CAD build for the part. Positions are in the model's coordinates, mm. Face numbers are marked on the shaded views. A direction names the side the tool comes from. Round coordinates to 2 decimals unless told otherwise and drop trailing zeros. Order: outer loops, then holes, each group sorted by start corner. A loop starts at its lowest first (then second) coordinate and runs counter-clockwise, first axis right, second up. Notation, with made-up numbers: (25.25, -23.75) -> (41.25, -23.75) arc R16 cw to (41.25, -1.75) -> close; hole circle Ø7 at (12, 26). An arc over 180 degrees is marked (long way). Return JSON: item names as keys, results as strings. Group by question number.
Q1. Cut at A-A (z = 6). Write the cut outline in (x, y).
Q2. Mould opens along Y. For the marked faces 1 and 2 say: +Y half, -Y half, draft (parallel to the pull), parting line (faces both ways), or undercut.
Q3. Probe line 1 along X through (y, z) = (10, 1.75); line 2 along X through (y, z) = (-25, 7.75). List the from-to ranges inside material, lowest first.
Q4. Flat gauge pins, fed straight in: pin 1 (1.8 mm diameter, centred on y = 28.5, z = 9.5, fed in from +X); pin 2 (8 mm diameter, centred on x = 26, y = -24, fed in from -Z); pin 3 (2 mm diameter, centred on y = 25, z = 7.5, fed in from +X); pin 4 (3 mm diameter, centred on x = -26, z = 12.5, fed in from +Y). Where does each tip first touch, or does it go through?
Q5. Which spindle directions (+Z, -Z, +X, -X, +Y, -Y) get a long thin tool onto all of the face, cutting with end or side? Do the marked faces 3 and 4. Say none if no direction does.
Q6. Cut at D-D (x = 28). Write the cut outline in (y, z).
Q7. Cut at B-B (x = -8). Write the cut outline in (y, z).
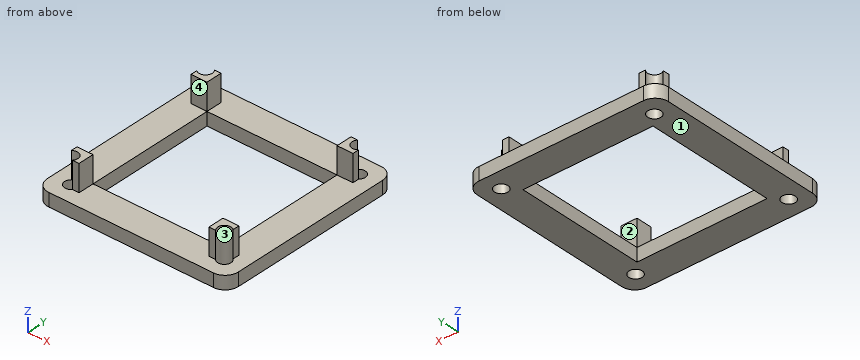
from build123d import *

# Parameters (mm, degrees)
PAD_DEPTH       = 5
SKETCH001_W     = 6
SKETCH001_H     = 6
PAD001_DEPTH    = 10
SKETCH002_W     = 49
SKETCH002_H     = 49
POCKET_DEPTH    = 5.001
SKETCH003_R     = 2.5
POCKET001_DEPTH = 15.001


with BuildPart() as part:
    # Sketch → Pad (new body)
    with BuildSketch(Plane.XY):
        with BuildLine():
            ThreePointArc((-31, 36), (-34.535534, 34.535534), (-36, 31))
            Line((-36, 31), (-36, -31))
            ThreePointArc((-36, -31), (-34.535534, -34.535534), (-31, -36))
            Line((-31, -36), (31, -36))
            ThreePointArc((31, -36), (34.535534, -34.535534), (36, -31))
            Line((36, -31), (36, 31))
            ThreePointArc((36, 31), (34.535534, 34.535534), (31, 36))
            Line((31, 36), (-31, 36))
        make_face()
    extrude(amount=PAD_DEPTH)

    # Sketch001 (on Face10 of Pad) → Pad001 (join)
    with BuildSketch(Plane.XY.offset(5)):
        with Locations((-27.5, 27.5)):
            Rectangle(SKETCH001_W, SKETCH001_H)
        with Locations((27.5, 27.5)):
            Rectangle(SKETCH001_W, SKETCH001_H)
        with Locations((27.5, -27.5)):
            Rectangle(SKETCH001_W, SKETCH001_H)
        with Locations((-27.5, -27.5)):
            Rectangle(SKETCH001_W, SKETCH001_H)
    extrude(amount=PAD001_DEPTH)

    # Sketch002 (on Face5 of Pad001) → Pocket (cut, through all)
    with BuildSketch(Plane.XY.offset(5)):
        Rectangle(SKETCH002_W, SKETCH002_H)
    extrude(amount=-POCKET_DEPTH, mode=Mode.SUBTRACT)

    # Sketch003 (on Face4 of Pocket) → Pocket001 (cut, through all)
    with BuildSketch(Plane(origin=(0, 0, 0), x_dir=(1, 0, 0), z_dir=(0, 0, -1))):
        with Locations((-28.849957, 28.849957)):
            Circle(SKETCH003_R)
        with Locations((28.849957, 28.849957)):
            Circle(SKETCH003_R)
        with Locations((28.849957, -28.849957)):
            Circle(SKETCH003_R)
        with Locations((-28.849957, -28.849957)):
            Circle(SKETCH003_R)
    extrude(amount=-POCKET001_DEPTH, mode=Mode.SUBTRACT)


solid = part.part
Solution:
{
 "1": {"outline": "(-30.5, -26.97) arc R2.5 cw to (-26.97, -30.5) -> (-24.5, -30.5) -> (-24.5, -24.5) -> (-30.5, -24.5) -> close; (-30.5, 24.5) -> (-24.5, 24.5) -> (-24.5, 30.5) -> (-26.97, 30.5) arc R2.5 cw to (-30.5, 26.97) -> close; (24.5, -30.5) -> (26.97, -30.5) arc R2.5 cw to (30.5, -26.97) -> (30.5, -24.5) -> (24.5, -24.5) -> close; (24.5, 24.5) -> (30.5, 24.5) -> (30.5, 26.97) arc R2.5 cw to (26.97, 30.5) -> (24.5, 30.5) -> close"},
 "2": {"face 1": "draft", "face 2": "undercut"},
 "3": {"line 1": "x = -36 to -24.5, 24.5 to 36", "line 2": "x = -30.5 to -24.5, 24.5 to 30.5"},
 "4": {"pin 1": "stops at x = 26.68", "pin 2": "stops at z = 0", "pin 3": "stops at x = 30.5", "pin 4": "stops at y = 30.5"},
 "5": {"face 3": "+Z, -Z", "face 4": "+Z, +X, -X"},
 "6": {"outline": "(-36, 0) -> (-31.2, 0) -> (-31.2, 5) -> (-36, 5) -> close; (-26.5, 0) -> (26.5, 0) -> (26.5, 15) -> (24.5, 15) -> (24.5, 5) -> (-24.5, 5) -> (-24.5, 15) -> (-26.5, 15) -> close; (31.2, 0) -> (36, 0) -> (36, 5) -> (31.2, 5) -> close"},
 "7": {"outline": "(-36, 0) -> (-24.5, 0) -> (-24.5, 5) -> (-36, 5) -> close; (24.5, 0) -> (36, 0) -> (36, 5) -> (24.5, 5) -> close"}
}
